Model file for the job. Use its own axes, mm. Coordinates: 2 decimals unless noted, no trailing zeros. Loops run counter-clockwise (first coordinate to the right, second up) from the corner with the lowest first, then second, coordinate; pieces in that order, holes last. Notation, with made-up numbers: (64, 55) -> (115, 55) arc R16 ccw to (115, 86) -> close; hole circle Ø8 at (-32.75, -33). An arc over 180 degrees is marked (long way). Use one line per item in the form item = value.
```python
from build123d import *

# Parameters (mm, degrees)
F0_R     = 7.2252124777
F1_DEPTH = 4.6355
F3_D     = 1.5875
F3_DEPTH = 4.064
F3_TIP   = 0.4769331164
F4_R     = 2.54


with BuildPart() as f1:
    # F0 (on Front) → F1 (new body)
    with BuildSketch(Plane.XZ):
        Circle(F0_R)
    extrude(amount=F1_DEPTH)

    # F3
    with Locations(Plane.XZ.offset(4.6355)):
        with Locations((0, 0)):
            Hole(F3_D / 2, depth=F3_DEPTH)
            with Locations((0, 0, -(F3_DEPTH + F3_TIP / 2))):  # 118° drill point
                Cone(0, F3_D / 2, F3_TIP, mode=Mode.SUBTRACT)

    # F4
    f4_edges = [f1.edges().sort_by_distance(p)[0] for p in [
        (-7.225212, -4.6355, 0),
    ]]
    fillet(f4_edges, radius=F4_R)


solid = f1.part
```
Q1. Band-saw the part on A-A, the plane y = -1.25. Write the cut outline in (x, z).
Result:
outline = circle Ø14.45 at (0, 0); hole circle Ø1.59 at (0, 0)
Q2. Wall check: line 1 along Z through (x, y) = (0, -1.6); line 2 along Z through (x, y) = (-0.5, -2); line 3 along Z through (x, y) = (-5, -2.75). Give the ranges that are in metal, low to high.
Result:
line_1 = -7.23 to -0.79, 0.79 to 7.23
line_2 = -7.21 to -0.62, 0.62 to 7.21
line_3 = -5.1 to 5.1
Q3. Band-saw the part on B-B, the plane y = -2.6. Write the cut outline in (x, z).
Result:
outline = circle Ø14.35 at (0, 0); hole circle Ø1.59 at (0, 0)
Q4. Mould opens along Z. For faces 1 (the face through (6.674, -1.033, -2.767)), 2 (the face through (0.172, -2.575, -0.775)), 3 (the face through (-0.1, 0, 0.1)) say: released by +Z, released by -Z, zero draft, split by the parting line, or undercut.
Result:
face_1 = split by the parting line
face_2 = undercut
face_3 = zero draft
Q5. Pin check, flat tips, straight feed: pin 1 Ø1 at (x, z) = (0, 0) entering from -Y (3 decimals); pin 2 Ø1.5 at (y, z) = (-2.5, 4.5) entering from +X; pin 3 Ø1 at (y, z) = (-3, 5) entering from +X; pin 4 Ø2 at (x, z) = (-5.5, 1.5) entering from -Y. Stop position of each tip, or through.
Result:
pin_1 = -0.395
pin_2 = 6.15
pin_3 = 5.49
pin_4 = -4.64
